from build123d import *
from build123d.topology import SkipClean

# Parameters (mm, degrees)
SKETCH1_R                                    = 30
BOSS_EXTRUDE3_DEPTH                          = 20
SKETCH1_3_R                                  = 30
SKETCH1_3_R_2                                = 20
BOSS_EXTRUDE4_DEPTH                          = 25
MIRROR1_AT_THE_SECOND_PLANE_COPY_1_SKETC_R   = 30
MIRROR1_AT_THE_SECOND_PLANE_COPY_1_DEPTH     = 20
MIRROR1_AT_THE_SECOND_PLANE_COPY_2_SKETC_R   = 30
MIRROR1_AT_THE_SECOND_PLANE_COPY_2_SKETC_R_2 = 20
MIRROR1_AT_THE_SECOND_PLANE_COPY_2_DEPTH     = 25


with BuildPart() as part:
    # Sketch1 → Boss-Extrude3 (new body)
    with BuildSketch(Plane.XY):
        with BuildLine():
            Line((-140, 100), (-140, 53.065996646))
            ThreePointArc((-140, 53.065996646), (-95.532624121, 41.569219382), (-76, 0))
            Line((-76, 0), (0, 0))
            Line((0, 0), (0, 70))
            ThreePointArc((0, 70), (-19.318516526, 84.823619098), (-10, 107.320508076))
            Line((-10, 107.320508076), (-10, 130))
            Line((-10, 130), (-50, 130))
            Line((-50, 130), (-50, 140))
            Line((-50, 140), (-100, 140))
            ThreePointArc((-100, 140), (-128.284271247, 128.284271247), (-140, 100))
        make_face()
        with Locations((-100, 100)):
            Circle(SKETCH1_R, mode=Mode.SUBTRACT)
    boss_extrude3 = extrude(amount=BOSS_EXTRUDE3_DEPTH)

    # Sketch1_3 → Boss-Extrude4 (add)
    with BuildSketch(Plane.XY):
        with Locations((-100, 100)):
            Circle(SKETCH1_3_R)
        with Locations((-100, 100)):
            Circle(SKETCH1_3_R_2, mode=Mode.SUBTRACT)
    boss_extrude4 = extrude(amount=BOSS_EXTRUDE4_DEPTH)



with BuildPart() as mirror1_1:
    # Mirror1: Boss-Extrude3, Boss-Extrude4 across plane
    add(boss_extrude3.mirror(Plane(origin=(0, 0, 0), x_dir=(0, 0, 1), z_dir=(1, 0, 0))))
    add(boss_extrude4.mirror(Plane(origin=(0, 0, 0), x_dir=(0, 0, 1), z_dir=(1, 0, 0))))


with BuildPart() as part_1:
    with SkipClean():  # the faces are left unmerged after this step: merging them gives an invalid solid
        add(part.part)

        add(mirror1_1.part)  # Mirror1 at the second plane merges Mirror1_1
        # Mirror1 at the second plane: Boss-Extrude3, Boss-Extrude4 across plane
        add(boss_extrude3.mirror(Plane.ZX))
        add(boss_extrude4.mirror(Plane.ZX))

    # Mirror1 at the second plane copy 1 sketc → Mirror1 at the second plane copy 1 (add)
    with SkipClean():  # the faces are left unmerged after this step: merging them gives an invalid solid
        with BuildSketch(Plane(origin=(0, 0, 0), x_dir=(-1, 0, 0), z_dir=(0, 0, 1))):
            with BuildLine():
                Line((-140, 100), (-140, 53.065996646))
                ThreePointArc((-140, 53.065996646), (-95.532624121, 41.569219382), (-76, 0))
                Line((-76, 0), (0, 0))
                Line((0, 0), (0, 70))
                ThreePointArc((0, 70), (-19.318516526, 84.823619098), (-10, 107.320508076))
                Line((-10, 107.320508076), (-10, 130))
                Line((-10, 130), (-50, 130))
                Line((-50, 130), (-50, 140))
                Line((-50, 140), (-100, 140))
                ThreePointArc((-100, 140), (-128.284271247, 128.284271247), (-140, 100))
            make_face()
            with Locations((-100, 100)):
                Circle(MIRROR1_AT_THE_SECOND_PLANE_COPY_1_SKETC_R, mode=Mode.SUBTRACT)
        extrude(amount=MIRROR1_AT_THE_SECOND_PLANE_COPY_1_DEPTH)

    # Mirror1 at the second plane copy 2 sketc → Mirror1 at the second plane copy 2 (add)
    with SkipClean():  # the faces are left unmerged after this step: merging them gives an invalid solid
        with BuildSketch(Plane(origin=(0, 0, 0), x_dir=(-1, 0, 0), z_dir=(0, 0, 1))):
            with Locations((-100, 100)):
                Circle(MIRROR1_AT_THE_SECOND_PLANE_COPY_2_SKETC_R)
            with Locations((-100, 100)):
                Circle(MIRROR1_AT_THE_SECOND_PLANE_COPY_2_SKETC_R_2, mode=Mode.SUBTRACT)
        extrude(amount=MIRROR1_AT_THE_SECOND_PLANE_COPY_2_DEPTH)


solid = part_1.part
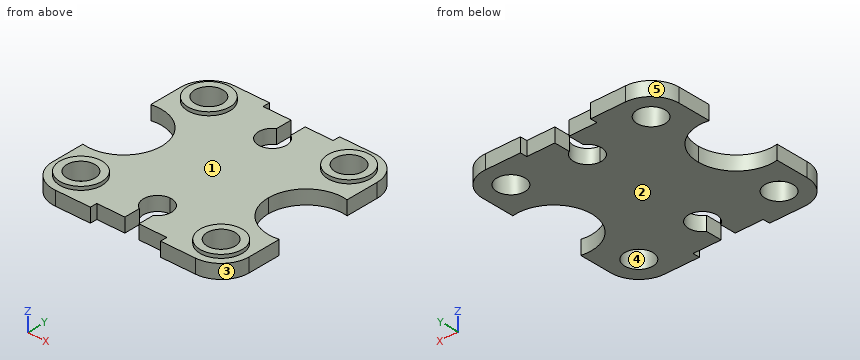
The listing builds one solid part. Answer for the finished solid, in the listing's coordinates (mm). Face numbers are marked on the shaded views. A direction names the side the tool comes from. Round coordinates to 2 decimals unless told otherwise and drop trailing zeros. Write each loop counter-clockwise with the first axis right and the second up, starting at its lowest first coordinate (ties: lowest second). Pieces come first, ordered by that corner, then holes. Notation, with made-up numbers: (7, 74.25) - (38, 74.25) arc R22 ccw to (38, 94.25) - close; hole circle Ø5 at (3.5, -6.75). An arc over 180 degrees is marked (long way). Use a Markdown table: item, result. Add a question column.
1. The part is cut by section C-C (z = 10.25). Give the number of separate pieces and of enclosed holes in the cut face, and give its area (3 significant figures).
2. A tool of negligible diameter and unlimited length cuts with its end or side. For the marked faces 1 and 2, from which of +Z, -Z, +X, -X, +Y, -Y can it reach the whole face along a straight path? Write none if from no direction.
3. For a pull along X with two mould halves and no side action, classify the marked faces 3, 4 and 5 as +X half, -X half, draft (parallel to the pull), parting line (faces both ways), or undercut.
4. The part is cut by section B-B (y = -110.5). Write down the section's boundary in (x, z).
5. The part is cut by section A-A (x = 108.5). Write down the section's boundary in (y, z), and give its area (3 significant figures).
6. Consider line 1 (Y direction, x = -99, z = 20.75); line 2 (X direction, y = -100, z = 15.5); line 3 (X direction, y = -82, z = 13). Determine where each line is inside the solid, lowest interval first.
7. The part is cut by section D-D (x = -41). Write down the section's boundary in (y, z), and give its area (3 significant figures).
8. Flat-ended cylindrical pins translate along their axes: P1, Ø1, axis at y = -49, z = 11, coming from the -X side; P2, Ø1.5, axis at y = -10, z = 7, coming from the -X side; P3, Ø5, axis at y = 134, z = 6, coming from the +X side. Find the tip coordinate at first contact, or state that the pin passes through.
Reported:
| question | item | result |
|---|---|---|
| 1 | separate pieces | 1 |
| 1 | enclosed holes | 4 |
| 1 | area | 55,300 mm^2 |
| 2 | face 1 | +Z |
| 2 | face 2 | -Z, +X, -X, +Y, -Y |
| 3 | face 3 | +X half |
| 3 | face 4 | undercut |
| 3 | face 5 | -X half |
| 4 | outline | (-138.6, 0) - (-117.02, 0) - (-117.02, 25) - (-128.1, 25) - (-128.1, 20) - (-138.6, 20) - close; (-82.98, 0) - (-10, 0) - (-10, 20) - (-71.9, 20) - (-71.9, 25) - (-82.98, 25) - close; (10, 0) - (82.98, 0) - (82.98, 25) - (71.9, 25) - (71.9, 20) - (10, 20) - close; (117.02, 0) - (138.6, 0) - (138.6, 20) - (128.1, 20) - (128.1, 25) - (117.02, 25) - close |
| 5 | outline | (-139.09, 0) - (-118.1, 0) - (-118.1, 25) - (-128.77, 25) - (-128.77, 20) - (-139.09, 20) - close; (-81.9, 0) - (-49.54, 0) - (-49.54, 20) - (-71.23, 20) - (-71.23, 25) - (-81.9, 25) - close; (49.54, 0) - (81.9, 0) - (81.9, 25) - (71.23, 25) - (71.23, 20) - (49.54, 20) - close; (118.1, 0) - (139.09, 0) - (139.09, 20) - (128.77, 20) - (128.77, 25) - (118.1, 25) - close |
| 5 | area | 2,350 mm^2 |
| 6 | line 1 | -129.98 to -119.97, -80.03 to -70.02, 70.02 to 80.03, 119.97 to 129.98 |
| 6 | line 2 | -140 to -120, -80 to -17.32, 17.32 to 80, 120 to 140 |
| 6 | line 3 | -140 to -108.72, -91.28 to -18.33, 18.33 to 91.28, 108.72 to 140 |
| 7 | outline | (-130, 0) - (130, 0) - (130, 20) - (-130, 20) - close |
| 7 | area | 5,200 mm^2 |
| 8 | P1 | x = -108.42 |
| 8 | P2 | x = -77.08 |
| 8 | P3 | x = 124.65 |
